Autodesk Fusion 360 part; units mm, degrees
sketch "Sketch1" plane through (0, 0, 0) normal (1, 0, 0) x (0, 1, 0)
  circle A0 centre (0, 0) radius 180
  circle A1 centre (0, 0) radius 300
  line L0 (0, 300) -> (830, 300)
  line L1 (830, 300) -> (830, 460)
  line L2 (830, 460) -> (1230, 460)
  line L3 (1230, 460) -> (1230, -40)
  line L4 (1230, -40) -> (1050, -40)
  line L5 (1050, 180) -> (450, 180)
  line L6 (450, 180) -> (450, -300)
  line L7 (450, -300) -> (0, -300)
  line L8 (1050, 180) -> (1050, -40)
  line L9 (1230, -40) -> (1410, -40)
  line L10 (1410, -40) -> (1410, 760)
  line L11 (1410, 760) -> (1230, 760)
  line L12 (1230, 760) -> (1230, -40)
  line L13 (1230, 760) -> (830, 460)
  line L14 (450, -300) -> (1050, -40)
  dimension "d1" = 360
  dimension "d2" = 600
  dimension "d3" = 800
  dimension "d4" = 180
  dimension "d5" = 180
  dimension "d6" = 450
  dimension "d7" = 600
  dimension "d8" = 160
  dimension "d9" = 120
  dimension "d10" = 220
  dimension "d11" = 400
  dimension "d12" = 480
extrude "Extrude1" add sketch "Sketch1" along normal mid plane 660 contours A1
extrude "Extrude2" add sketch "Sketch1" along normal mid plane 540 contours A1 L0 L1 L2 L3 L4 L5 L6 L7 L8 L12
extrude "Extrude3" add sketch "Sketch1" along normal mid plane 120 contours L2 L12 L13
extrude "Extrude4" add sketch "Sketch1" along normal mid plane 920 contours L3 L9 L10 L11 L12
extrude "Extrude5" add sketch "Sketch1" along normal mid plane 200 contours L5 L6 L8 L14
fillet "Fillet1" radius 200 2 edges at (460, 1320, 760) (-460, 1320, 760)
sketch "Sketch2" plane through (0, 0, 300) normal (0, 0, 1) x (-1, 0, 0)
  line L0 (270, 0) -> (-270, 0)
  line L1 (-270, 0) -> (-270, -830)
  line L2 (-270, -830) -> (270, -830)
  line L3 (270, -830) -> (270, 0)
  line L4 (50, 314.5637) -> (-50, 314.5637)
  line L5 (-50, 314.5637) -> (-50, -314.5637)
  line L6 (-50, -314.5637) -> (50, -314.5637)
  line L7 (50, -314.5637) -> (50, 314.5637)
  line L8 (50, 314.5637) -> (-50, -314.5637) construction
  line L9 (-50, 314.5637) -> (50, -314.5637) construction
  point P0 (330, 300)
  point P1 (-330, 300)
  dimension "d25" = 100
  dimension "d26" = 280
  dimension "d27" = 280
extrude "Extrude6" cut sketch "Sketch2" against normal blind 1200 contours L0 L5 L6 L7 | L0 L4 L5 L7
hole "Hole1" at (260, 1230, 560) direction (0, 1, 0) diameter 160 end through all
mirror "Mirror1" about plane through (0, 0, 0) normal (1, 0, 0) of "Hole1"
Here's how the part is built. I have some questions about the finished solid (model axes, mm). A direction names the side the tool comes from. Round coordinates to 2 decimals unless told otherwise and drop trailing zeros. Write each loop counter-clockwise with the first axis right and the second up, starting at its lowest first coordinate (ties: lowest second). Pieces come first, ordered by that corner, then holes. Notation, with made-up numbers: (45.25, 41) -> (49.25, 41) arc R22 ccw to (49.25, 51) -> close; hole circle Ø11 at (-29.75, 41). An arc over 180 degrees is marked (long way). One line per item, written item: value.
1) I'm going to push flat-ended pins straight in: pin 1 Ø5 at (x, y) = (53, 1059) entering from +Z (3 decimals); pin 2 Ø1 at (x, z) = (118, 388) entering from -Y; pin 3 Ø1 at (x, y) = (113, 619.5) entering from +Z. Where does each tip first touch, or does it pass through?
Filled sheet:
pin 1: stops at z = 633.625
pin 2: stops at y = 830
pin 3: stops at z = 300
2) Suppose I cut it at A-A on z = 0. Give the number of separate pieces and of enclosed holes in the cut face, plus the area to 3 significant figures.
Filled sheet:
separate pieces: 3
enclosed holes: 0
area: 597,000 mm2
3) For faces 4 (the face through (-64, 228, -300)), 5 (the face through (-186, 1050, 72)), 6 (the face through (-6, 1267, -40)), 7 (the face through (-60, 1116, 545)), which set-ups out of +Z, -Z, +X, -X, +Y, -Y let a thin tool reach every point of the face, with its end or its side?
Filled sheet:
face 4: -Z, +X, -X, +Y, -Y
face 5: -Z, -X
face 6: -Z, +X, -X, +Y
face 7: +Z, -X, -Y
4) Suppose I cut it at B-B on y = 278. List the corners of the cut face in (x, z) for me.
Filled sheet:
outline: (-330, -112.77) -> (-270, -112.77) -> (-270, -300) -> (-50, -300) -> (-50, 300) -> (-270, 300) -> (-270, 112.77) -> (-330, 112.77) -> close; (50, -300) -> (270, -300) -> (270, -112.77) -> (330, -112.77) -> (330, 112.77) -> (270, 112.77) -> (270, 300) -> (50, 300) -> close
5) We'd pull the mould along X, two halves only. Please class faces 1 (the face through (1, 314.564, 4)), 2 (the face through (184, 754, 180)), 3 (the face through (60, 1116, 545)): released by +X, released by -X, zero draft, split by the parting line, or undercut.
Filled sheet:
face 1: undercut
face 2: zero draft
face 3: released by +X
6) Suppose I cut it at D-D on z = 517. List the corners of the cut face in (x, y) for me.
Filled sheet:
outline: (-460, 1230) -> (-327.46, 1230) -> (-327.46, 1410) -> (-460, 1410) -> close; (-192.54, 1230) -> (-60, 1230) -> (-60, 906) -> (60, 906) -> (60, 1230) -> (192.54, 1230) -> (192.54, 1410) -> (-192.54, 1410) -> close; (327.46, 1230) -> (460, 1230) -> (460, 1410) -> (327.46, 1410) -> close
7) Suppose I cut it at C-C on z = 350.5. List the corners of the cut face in (x, y) for me.
Filled sheet:
outline: (-460, 1230) -> (-270, 1230) -> (-270, 830) -> (270, 830) -> (270, 1230) -> (460, 1230) -> (460, 1410) -> (-460, 1410) -> close
8) If I drill on line 1 (X direction, y = 1365, z = 560); line 2 (Y direction, x = -130, z = 0); line 3 (Z direction, x = -260, y = 1267), over which ranges is the centre line in solid material (lowest first)? Write a range as [from, to].
Filled sheet:
line 1: x = [-460, -340], [-180, 180], [340, 460]
line 2: y = [-300, -180], [180, 450], [1050, 1410]
line 3: z = [-40, 480], [640, 760]
